Input: part model. Units: mm. Frame: model coordinates. Face numbers are marked on the shaded views. Round coordinates to 2 decimals unless told otherwise and drop trailing zeros. Loops run counter-clockwise (first coordinate to the right, second up) from the corner with the lowest first, then second, coordinate; pieces in that order, holes last. Notation, with made-up numbers: M 83.25,-23.5 L 129.25,-23.5 A27 cw 129.25,1.5 Z; hole C 4.5,-34.5 d5. An arc over 180 degrees is marked long. Use one line per item in the form item = value. Start each with the question number.
Q1. Mould query, pull axis Z, two halves, no side actions, for the marked faces 1 and 2. Classes: pulls with the +Z half, pulls with the -Z half, needs draft (parallel to the pull), parting line crosses it, or undercut.
Q2. Section query C-C, the plane y = 23.5. Output: boundary loops of the cut face in (x, z).
Q3. First-contact query: P1, Ø1.1, axis at y = 42.5, z = -4, coming from the +X side; P2, Ø1.1, axis at y = 47, z = -4.5, coming from the -X side; P3, Ø0.5, axis at y = 41.5, z = -4, coming from the -X side. Flat tips, straight axial feed; report the tip coordinate or a pass-through.
Q4. Section query D-D, the plane y = 44. Output: boundary loops of the cut face in (x, z).
Q5. Section query A-A, the plane x = 0. Output: boundary loops of the cut face in (y, z), and give its area (3 significant figures).
Q6. Ray query, line 1 along Y through (x, z) = (-2.5, 3.75); line 2 along X through (y, z) = (12, 0); line 3 along Y through (x, z) = (4.25, 2.5). Return the intervals inside material, ascending.
Q7. Section query B-B, the plane z = 0. Output: boundary loops of the cut face in (x, y), and give its area (4 significant figures).
```python
from build123d import *

# Parameters (mm, degrees)
ESQUISSE1_R                  = 5
ESQUISSE1_R_2                = 3
BOSS_EXTRU_1_DEPTH           = 48.5
ENL_V_MAT_EXTRU_1_DEPTH      = 5
ENL_V_MAT_EXTRU_2_REACH      = 51.901
ENL_V_MAT_EXTRU_2_END_RADIUS = 3
ESQUISSE3_R                  = 1
ESQUISSE4_R                  = 5
ESQUISSE4_R_2                = 4
ENL_V_MAT_EXTRU_3_DEPTH      = 1
ESQUISSE6_R                  = 5
ESQUISSE6_R_2                = 4
ENL_V_MAT_EXTRU_5_DEPTH      = 1
ENL_V_MAT_EXTRU_4_REACH      = 51.013


with BuildPart() as part:
    # Esquisse1 → Boss.-Extru.1 (new body)
    with BuildSketch(Plane(origin=(0, 0, 0), x_dir=(1, 0, 0), z_dir=(0, 1, 0))):
        with Locations(Location((0, 0, 0), (0, 0, 90))):
            Circle(ESQUISSE1_R)
        with Locations(Location((0, 0, 0), (0, 0, 90))):
            Circle(ESQUISSE1_R_2, mode=Mode.SUBTRACT)
    extrude(amount=BOSS_EXTRU_1_DEPTH)

    # Esquisse2 → Enlèv. mat.-Extru.1 (cut)
    with BuildSketch(Plane.XZ):
        with BuildLine():
            Line((-1.5, -4.769696007), (1.5, -4.769696007))
            ThreePointArc((1.5, -4.769696007), (0, -5), (-1.5, -4.769696007))
        make_face()
        with BuildLine():
            Line((-3.38067791, 3.683886109), (-4.88067791, 1.085809898))
            ThreePointArc((-4.88067791, 1.085809898), (-4.330127019, 2.5), (-3.38067791, 3.683886109))
        make_face()
        with BuildLine():
            Line((4.88067791, 1.085809898), (3.38067791, 3.683886109))
            ThreePointArc((3.38067791, 3.683886109), (4.330127019, 2.5), (4.88067791, 1.085809898))
        make_face()
    extrude(amount=-ENL_V_MAT_EXTRU_1_DEPTH, mode=Mode.SUBTRACT)

    # Enlèv. mat.-Extru.2: up to this cylinder (the profile starts outside it)
    enl_v_mat_extru_2_end = Plane(origin=(0, 2.5, 0), z_dir=(0, -1, 0)) * Cylinder(ENL_V_MAT_EXTRU_2_END_RADIUS, 110.802, mode=Mode.PRIVATE)
    # Esquisse3 → Enlèv. mat.-Extru.2 (cut, up to the surface)
    with BuildSketch(Plane(origin=(4.13067791, 0, 2.384848004), x_dir=(0.49999999999999223, 0, -0.8660254037844431), z_dir=(0.8660254037844431, 0, 0.49999999999999223)), mode=Mode.PRIVATE) as enl_v_mat_extru_2_sk1:
        with Locations((0, 2.5)):
            Circle(ESQUISSE3_R)
    enl_v_mat_extru_2_tool1 = extrude(enl_v_mat_extru_2_sk1.sketch, amount=-ENL_V_MAT_EXTRU_2_REACH, mode=Mode.PRIVATE) - enl_v_mat_extru_2_end
    add(enl_v_mat_extru_2_tool1.solids().sort_by_distance((4.130678, 2.5, 2.384848))[0], mode=Mode.SUBTRACT)

    # Esquisse4 → Enlèv. mat.-Extru.3 (cut)
    with BuildSketch(Plane(origin=(0, 39.5, 0), x_dir=(-1, 0, 0), z_dir=(0, -1, 0))):
        with Locations(Location((0, 0, 0), (0, 0, 90))):
            Circle(ESQUISSE4_R)
        with Locations(Location((0, 0, 0), (0, 0, 90))):
            Circle(ESQUISSE4_R_2, mode=Mode.SUBTRACT)
    extrude(amount=-ENL_V_MAT_EXTRU_3_DEPTH, mode=Mode.SUBTRACT)

    # Esquisse6 → Enlèv. mat.-Extru.5 (cut)
    with BuildSketch(Plane(origin=(0, 43.5, 0), x_dir=(-1, 0, 0), z_dir=(0, -1, 0))):
        with Locations(Location((0, 0, 0), (0, 0, 90))):
            Circle(ESQUISSE6_R)
        with Locations(Location((0, 0, 0), (0, 0, 90))):
            Circle(ESQUISSE6_R_2, mode=Mode.SUBTRACT)
    extrude(amount=-ENL_V_MAT_EXTRU_5_DEPTH, mode=Mode.SUBTRACT)

    # Enlèv. mat.-Extru.4: up to this face of the body (flat: up to its plane)
    enl_v_mat_extru_4_end = Plane(part.part.faces().sort_by_distance((0, 39.5, 4.858578644))[0])
    # Esquisse5 → Enlèv. mat.-Extru.4 (cut, up to the picked face)
    with BuildSketch(Plane(origin=(0, 48.5, 0), x_dir=(1, 0, 0), z_dir=(0, 1, 0)), mode=Mode.PRIVATE) as enl_v_mat_extru_4_sk1:
        with BuildLine():
            Line((-1.5, 3.769696007), (1.5, 3.769696007))
            Line((1.5, 3.769696007), (1.5, 4.769696007))
            ThreePointArc((1.5, 4.769696007), (0, 5), (-1.5, 4.769696007))
            Line((-1.5, 4.769696007), (-1.5, 3.769696007))
        make_face()
    enl_v_mat_extru_4_tool1 = split(extrude(enl_v_mat_extru_4_sk1.sketch, amount=-ENL_V_MAT_EXTRU_4_REACH, mode=Mode.PRIVATE), bisect_by=enl_v_mat_extru_4_end, keep=Keep.BOTH, mode=Mode.PRIVATE)
    add(enl_v_mat_extru_4_tool1.solids().sort_by(Axis((0, 48.5, -4.348853), (0, -1, 0)))[0], mode=Mode.SUBTRACT)

    # Chanfrein1: read off the stored shape, not the designer's step
    # Chanfrein1 outline → Chanfrein1 (revolve, cut)
    with BuildSketch(Plane.XY):
        Polygon((5, 0.5), (4.5, 0), (5, 0), align=None)
        Polygon((4.5, 48.5), (5, 48), (5, 48.5), align=None)
    revolve(axis=Axis((0, 0, 0), (0, 1, 0)), mode=Mode.SUBTRACT)


solid = part.part
```
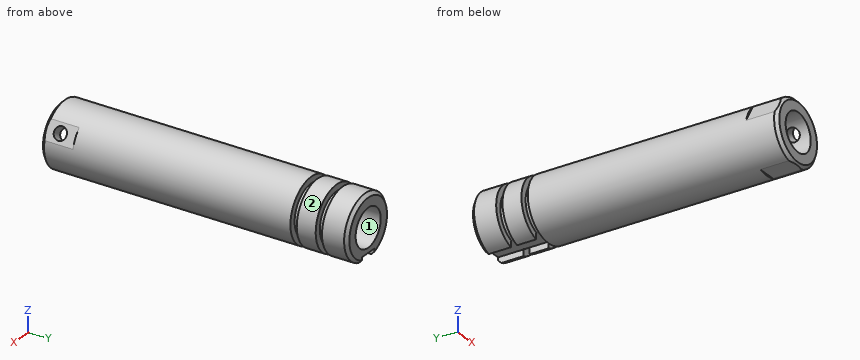
Results found:
q1.face_1 = undercut
q1.face_2 = parting line crosses it
q2.outline = C 0,0 d10; hole C 0,0 d6
q3.P1 = 3.62
q3.P2 = -3.07
q3.P3 = -3.31
q4.outline = M -1.34,-3.77 L 1.34,-3.77 A4 ccw long Z; hole C 0,0 d6
q5.outline = M 0,-4.5 L 0.27,-4.77 L 5,-4.77 L 5,-5 L 39.5,-5 L 39.5,-3.77 L 48.5,-3.77 L 48.5,-3 L 0,-3 Z; M 0,3 L 48.5,3 L 48.5,4.5 L 48,5 L 44.5,5 L 44.5,4 L 43.5,4 L 43.5,5 L 40.5,5 L 40.5,4 L 39.5,4 L 39.5,5 L 0.5,5 L 0,4.5 Z
q5.area = 179 mm²
q6.line_1 = 0.01 to 39.5, 40.5 to 43.5, 44.5 to 48.49
q6.line_2 = -5 to -3, 3 to 5
q6.line_3 = 5 to 39.5, 40.5 to 43.5, 44.5 to 48.07
q7.outline = M -5,0.5 L -4.5,0 L -3,0 L -3,48.5 L -4.5,48.5 L -5,48 L -5,44.5 L -4,44.5 L -4,43.5 L -5,43.5 L -5,40.5 L -4,40.5 L -4,39.5 L -5,39.5 Z; M 3,0 L 4.5,0 L 5,0.5 L 5,39.5 L 4,39.5 L 4,40.5 L 5,40.5 L 5,43.5 L 4,43.5 L 4,44.5 L 5,44.5 L 5,48 L 4.5,48.5 L 3,48.5 Z
q7.area = 189.5 mm²
